CAD build for the part. Positions are in the model's coordinates, mm. Face numbers are marked on the shaded views. A direction names the side the tool comes from. Coordinates: 2 decimals unless noted, no trailing zeros. Order: outer loops, then holes, each group sorted by start corner. A loop starts at its lowest first (then second) coordinate and runs counter-clockwise, first axis right, second up. Notation, with made-up numbers: (-28, -36.5) - (-23, -36.5) arc R20 cw to (-23, -21.5) - close; hole circle Ø10 at (36.5, 68.25). An arc over 180 degrees is marked (long way). Return JSON: item names as keys, results as strings.
from build123d import *

# Parameters (mm, degrees)
SKETCH_2_W        = 28
SKETCH_2_H        = 28
EXTRUDE_3_DEPTH   = 12
EXTRUDE_3_2_DEPTH = 12
EXTRUDE_3_3_DEPTH = 12
SKETCH_2_3_W      = 9
SKETCH_2_3_H      = 28
SKETCH_2_3_W_2    = 28
EXTRUDE_4_DEPTH   = 3
FILLET_1_R        = 1


with BuildPart() as part:
    # Sketch 2 → Extrude 3 (new body)
    with BuildSketch(Plane(origin=(0, 0, 0), x_dir=(1, 0, 0), z_dir=(0, 1, 0))):
        with Locations((-37, 0)):
            Rectangle(SKETCH_2_W, SKETCH_2_H)
    extrude(amount=-EXTRUDE_3_DEPTH)



with BuildPart() as body_2:
    # Sketch 2 → Extrude 3 2 (new body)
    with BuildSketch(Plane(origin=(0, 0, 0), x_dir=(1, 0, 0), z_dir=(0, 1, 0))):
        Rectangle(SKETCH_2_W, SKETCH_2_H)
    extrude(amount=-EXTRUDE_3_2_DEPTH)


with BuildPart() as body_3:
    # Sketch 2 → Extrude 3 3 (new body)
    with BuildSketch(Plane(origin=(0, 0, 0), x_dir=(1, 0, 0), z_dir=(0, 1, 0))):
        with Locations((37, 0)):
            Rectangle(SKETCH_2_W, SKETCH_2_H)
    extrude(amount=-EXTRUDE_3_3_DEPTH)


with BuildPart() as part_1:
    add(part.part)

    add(body_2.part)  # Extrude 4 merges body 2

    add(body_3.part)  # Extrude 4 merges body 3
    # Sketch 2_3 → Extrude 4 (add)
    with BuildSketch(Plane(origin=(0, 0, 0), x_dir=(1, 0, 0), z_dir=(0, 1, 0))):
        with Locations((-18.5, 0)):
            Rectangle(SKETCH_2_3_W, SKETCH_2_3_H)
        with Locations((-37, 0)):
            Rectangle(SKETCH_2_3_W_2, SKETCH_2_3_H)
        Rectangle(SKETCH_2_3_W_2, SKETCH_2_3_H)
        with Locations((18.5, 0)):
            Rectangle(SKETCH_2_3_W, SKETCH_2_3_H)
        with Locations((37, 0)):
            Rectangle(SKETCH_2_3_W_2, SKETCH_2_3_H)
    extrude(amount=EXTRUDE_4_DEPTH)

    # Fillet 1
    fillet_1_edges = [part_1.edges().sort_by_distance(p)[0] for p in [
        (-37, -12, -14),
        (-51, -12, 0),
        (0, 3, -14),
        (51, -4.5, -14),
        (-18.5, 0, 14),
        (51, 3, 0),
        (51, -4.5, 14),
        (-51, 3, 0),
        (0, 3, 14),
        (-18.5, 0, -14),
        (-37, -12, 14),
        (18.5, 0, -14),
        (18.5, 0, 14),
        (14, 0, 0),
        (14, -6, -14),
        (0, -12, 14),
        (14, -6, 14),
        (-14, -12, 0),
        (-14, -6, 14),
        (-14, -6, -14),
        (14, -12, 0),
        (0, -12, -14),
        (-14, 0, 0),
        (37, -12, 14),
        (23, -12, 0),
        (23, -6, 14),
        (23, -6, -14),
        (51, -12, 0),
        (37, -12, -14),
        (23, 0, 0),
        (-23, -12, 0),
        (-23, 0, 0),
        (-23, -6, 14),
        (-51, -4.5, 14),
        (-51, -4.5, -14),
        (-23, -6, -14),
    ]]
    fillet(fillet_1_edges, radius=FILLET_1_R)


solid = part_1.part
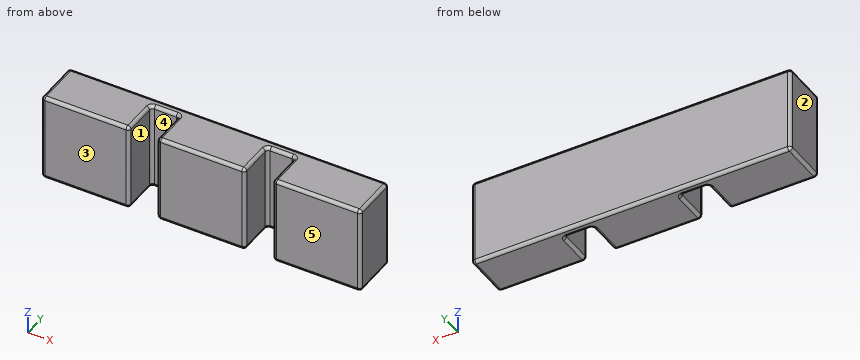
Item 1: Band-saw the part on A-A, the plane y = -8.25. List the corners of the cut face in (x, z), then the cut area to 3 significant figures.
Findings below:
{"outline": "(-51, -13) arc R1 ccw to (-50, -14) - (-24, -14) arc R1 ccw to (-23, -13) - (-23, 13) arc R1 ccw to (-24, 14) - (-50, 14) arc R1 ccw to (-51, 13) - close; (-14, -13) arc R1 ccw to (-13, -14) - (13, -14) arc R1 ccw to (14, -13) - (14, 13) arc R1 ccw to (13, 14) - (-13, 14) arc R1 ccw to (-14, 13) - close; (23, -13) arc R1 ccw to (24, -14) - (50, -14) arc R1 ccw to (51, -13) - (51, 13) arc R1 ccw to (50, 14) - (24, 14) arc R1 ccw to (23, 13) - close", "area": "2,350 mm²"}
Item 2: Which spindle directions (+Z, -Z, +X, -X, +Y, -Y) get a long thin tool onto all of the face, cutting with end or side? Do the marked faces 4 and 5. Say none if no direction does.
Findings below:
{"face 4": "+Z, -Z, -Y", "face 5": "+Z, -Z, +X, -X, -Y"}
Item 3: Mould opens along X. For the marked faces 1, 2 and 3 say: released by +X, released by -X, zero draft, split by the parting line, or undercut.
Findings below:
{"face 1": "undercut", "face 2": "released by -X", "face 3": "zero draft"}
Item 4: Band-saw the part on B-B, the plane x = 16.5. List the corners of the cut face in (y, z).
Findings below:
{"outline": "(0, -13) arc R1 ccw to (1, -14) - (2, -14) arc R1 ccw to (3, -13) - (3, 13) arc R1 ccw to (2, 14) - (1, 14) arc R1 ccw to (0, 13) - close"}
Item 5: Band-saw the part on C-C, the plane z = 0.5. List the corners of the cut face in (x, y).
Findings below:
{"outline": "(-51, -11) arc R1 ccw to (-50, -12) - (-24, -12) arc R1 ccw to (-23, -11) - (-23, -1) arc R1 cw to (-22, 0) - (-15, 0) arc R1 cw to (-14, -1) - (-14, -11) arc R1 ccw to (-13, -12) - (13, -12) arc R1 ccw to (14, -11) - (14, -1) arc R1 cw to (15, 0) - (22, 0) arc R1 cw to (23, -1) - (23, -11) arc R1 ccw to (24, -12) - (50, -12) arc R1 ccw to (51, -11) - (51, 2) arc R1 ccw to (50, 3) - (-50, 3) arc R1 ccw to (-51, 2) - close"}
Item 6: Wall check: L1, parallel to X at y = -9, z = 10.75; L2, parallel to Y at x = -16, z = -3.25. Give the ranges that are in metal, low to high. Write a range as [from, to].
Findings below:
{"L1": "x = [-51, -23], [-14, 14], [23, 51]", "L2": "y = [0, 3]"}
Item 7: Drop a flat-ended pin along its axis: P1, Ø3.5, axis at x = 18.5, z = 0.5, coming from the -Y side. Give the stop position or say it passes through.
Findings below:
{"P1": "stops at y = 0"}
